```python
from build123d import *

# Parameters (mm, degrees)
SKETCH001_W          = 167.35
SKETCH001_H          = 77.5
SKETCH001_W_2        = 91
SKETCH001_H_2        = 58.3
PAD_DEPTH            = 2.5
SKETCH_R             = 1.58
POCKET_DEPTH         = 0.001
POCKET_DEPTH_BACK    = 2.501
SKETCH002_W          = 96.2
SKETCH002_H          = 62.3
SKETCH002_W_2        = 91
SKETCH002_H_2        = 58.3
PAD001_DEPTH         = 37
SKETCH003_W          = 96.2
SKETCH003_H          = 62.3
PAD002_DEPTH         = 1.5
SKETCH004_W          = 19.5
SKETCH004_H          = 21
POCKET001_DEPTH      = 9.601
SKETCH005_W          = 53.9
SKETCH005_H          = 37
POCKET002_DEPTH      = 48.5
SKETCH007_W          = 16
SKETCH007_H          = 11.1
SKETCH007_W_2        = 9.8
SKETCH007_H_2        = 8.8
POCKET003_DEPTH      = 38.751
FILLET_R             = 2
POCKET004_DEPTH      = 377.854265
POCKET004_DEPTH_BACK = 418.854265


with BuildPart() as part:
    # Sketch001 → Pad (new body)
    with BuildSketch(Plane.XY):
        Rectangle(SKETCH001_W, SKETCH001_H)
        Rectangle(SKETCH001_W_2, SKETCH001_H_2, mode=Mode.SUBTRACT)
    extrude(amount=PAD_DEPTH)

    # Sketch → Pocket (cut, two sides)
    with BuildSketch(Plane.XY) as pocket_sk:
        with Locations((-76.675, -31.75)):
            Circle(SKETCH_R)
        with Locations((-76.675, 31.75)):
            Circle(SKETCH_R)
        with Locations((76.675, 31.75)):
            Circle(SKETCH_R)
        with Locations((76.675, -31.75)):
            Circle(SKETCH_R)
    extrude(amount=-POCKET_DEPTH, mode=Mode.SUBTRACT)
    extrude(pocket_sk.sketch, amount=POCKET_DEPTH_BACK, mode=Mode.SUBTRACT)

    # Sketch002 → Pad001 (join)
    with BuildSketch(Plane.XY.offset(2.5)):
        with Locations((-0.4, 1)):
            Rectangle(SKETCH002_W, SKETCH002_H)
        Rectangle(SKETCH002_W_2, SKETCH002_H_2, mode=Mode.SUBTRACT)
    extrude(amount=PAD001_DEPTH)

    # Sketch003 → Pad002 (join)
    with BuildSketch(Plane.XY.offset(39.5)):
        with Locations((-0.4, 1)):
            Rectangle(SKETCH003_W, SKETCH003_H)
        with BuildLine():
            ThreePointArc((0, 11.892024), (-16.168632, 3.339331), (-18.197313, -14.839164))
            ThreePointArc((-18.197313, -14.839164), (-15.316051, -16.091394), (-14.063821, -13.210132))
            ThreePointArc((0, 7.449109), (-12.495952, 0.839146), (-14.063821, -13.210132))
            ThreePointArc((0, 7.449109), (2.221458, 9.670566), (0, 11.892024))
        make_face(mode=Mode.SUBTRACT)
        with BuildLine():
            ThreePointArc((-0.208963, -6.182796), (15.203911, -11.065575), (21.251521, 3.928579))
            ThreePointArc((25.403758, 5.50922), (22.537319, 6.795018), (21.251521, 3.928579))
            ThreePointArc((-4.071455, -8.378395), (17.097581, -15.084718), (25.403758, 5.50922))
            ThreePointArc((-0.208963, -6.182796), (-3.238008, -5.349349), (-4.071455, -8.378395))
        make_face(mode=Mode.SUBTRACT)
        with BuildLine():
            ThreePointArc((31.656498, 5.917571), (17.941279, 12.959928), (14.941672, -2.163047))
            ThreePointArc((11.627583, -5.122155), (14.764181, -5.299645), (14.941672, -2.163047))
            ThreePointArc((36.034044, 6.676909), (16.007515, 16.959935), (11.627583, -5.122155))
            ThreePointArc((31.656498, 5.917571), (34.22494, 4.108467), (36.034044, 6.676909))
        make_face(mode=Mode.SUBTRACT)
        with BuildLine():
            ThreePointArc((-4.63181, 21.445734), (-29.723459, 6.034298), (-24.464471, -22.938901))
            ThreePointArc((-24.464471, -22.938901), (-21.322913, -22.957951), (-21.303863, -19.816393))
            ThreePointArc((-4.849326, 17.008146), (-25.66708, 4.221761), (-21.303863, -19.816393))
            ThreePointArc((-4.849326, 17.008146), (-2.521774, 19.118182), (-4.63181, 21.445734))
        make_face(mode=Mode.SUBTRACT)
    extrude(amount=PAD002_DEPTH)

    # Sketch004 → Pocket001 (cut, through all)
    with BuildSketch(Plane.XZ.offset(-29.15)):
        with Locations((-40.015, 10.5)):
            Rectangle(SKETCH004_W, SKETCH004_H)
    extrude(amount=-POCKET001_DEPTH, mode=Mode.SUBTRACT)

    # Sketch005 → Pocket002 (cut)
    with BuildSketch(Plane.YZ):
        with Locations((0, 21)):
            Rectangle(SKETCH005_W, SKETCH005_H)
    extrude(amount=POCKET002_DEPTH, mode=Mode.SUBTRACT)

    # Sketch007 → Pocket003 (cut, through all)
    with BuildSketch(Plane(origin=(0, 0, 0), x_dir=(-1, 0, 0), z_dir=(0, 1, 0))):
        with BuildLine():
            Line((-15.6, 2.5), (-15.6, 10.1))
            ThreePointArc((-7.8, 10.1), (-11.7, 14), (-15.6, 10.1))
            Line((-7.8, 2.5), (-7.8, 10.1))
            Line((-15.6, 2.5), (-7.8, 2.5))
        make_face()
        with Locations((10.52, 8.05)):
            Rectangle(SKETCH007_W, SKETCH007_H)
        with Locations((32, 6.9)):
            Rectangle(SKETCH007_W_2, SKETCH007_H_2)
    extrude(amount=-POCKET003_DEPTH, mode=Mode.SUBTRACT)

    # Fillet
    fillet_edges = [part.edges().sort_by_distance(p)[0] for p in [
        (47.7, -30.15, 21),
        (47.7, 32.15, 21),
        (-48.5, 32.15, 30.25),
        (-48.5, -30.15, 21),
        (-83.675, -38.75, 1.25),
        (-83.675, 38.75, 1.25),
        (83.675, 38.75, 1.25),
        (83.675, -38.75, 1.25),
        (-49.765, 38.75, 1.25),
        (-30.265, 38.75, 1.25),
        (-45.5, 29.15, 1.25),
    ]]
    fillet(fillet_edges, radius=FILLET_R)

    # Sketch008 → Pocket004 (cut, two sides)
    with BuildSketch(Plane.XY) as pocket004_sk:
        with BuildLine():
            ThreePointArc((-56.80108, -10.00872), (-57.069005, 12.779324), (-77.692091, 22.477522))
            ThreePointArc((-77.692091, 22.477522), (-82.034221, 16.942851), (-76.49955, 12.60072))
            ThreePointArc((-65.292956, -4.82592), (-65.436679, 7.398302), (-76.49955, 12.60072))
            ThreePointArc((-65.292956, -4.82592), (-63.638418, -11.663258), (-56.80108, -10.00872))
        make_face()
        with BuildLine():
            ThreePointArc((-76.93054, -4.199269), (-74.278684, -23.506721), (-56.126644, -30.599921))
            ThreePointArc((-56.126644, -30.599921), (-53.792985, -27.379186), (-57.01372, -25.045527))
            ThreePointArc((-71.737576, -6.360594), (-69.860738, -20.025349), (-57.01372, -25.045527))
            ThreePointArc((-71.737576, -6.360594), (-73.253395, -2.68345), (-76.93054, -4.199269))
        make_face()
    pocket004 = extrude(amount=-POCKET004_DEPTH, mode=Mode.SUBTRACT) + extrude(pocket004_sk.sketch, amount=POCKET004_DEPTH_BACK, mode=Mode.SUBTRACT)

    # Mirrored: Pocket004 across Sketch008 V_Axis
    add(pocket004.mirror(Plane(origin=(0, 0, 0), x_dir=(0, 0, 1), z_dir=(1, 0, 0))), mode=Mode.SUBTRACT)


solid = part.part
```
Could you check a few things on this model? Use its own coordinates, in mm. A direction names the side the tool comes from. Round coordinates to 2 decimals unless told otherwise and drop trailing zeros. Loops run counter-clockwise (first coordinate to the right, second up) from the corner with the lowest first, then second, coordinate; pieces in that order, holes last. Notation, with made-up numbers: (-6.75, 76) -> (0.25, 76) arc R27 ccw to (0.25, 110) -> close; hole circle Ø11 at (-28.5, 60). An arc over 180 degrees is marked (long way). Put each result on its own line as item: value.
Q1. I want a section at B-B on x = -40. Write out the boundary of the cut face in (y, z), and give its area (3 significant figures).
Checks:
outline: (-38.75, 0) -> (-29.15, 0) -> (-29.15, 39.5) -> (29.15, 39.5) -> (29.15, 21) -> (32.15, 21) -> (32.15, 41) -> (-30.15, 41) -> (-30.15, 2.5) -> (-38.75, 2.5) -> close
area: 210 mm2
Q2. Which directions (+Z, -Z, +X, -X, +Y, -Y) give clear straight access to the entire face, cutting with the end or side of a thin tool? Please do faces 3 (the cylindrical face through (16.787, -15.227, 40.24)), 4 (the flat face through (-1, 29.15, 19)).
Checks:
face 3: +Z, -Z
face 4: -Z
Q3. For pin 1 Ø1.8 at (x, z) = (46, 13) entering from +Y; pin 2 Ø0.8 at (y, z) = (-30, 7.5) entering from -X; pin 3 Ø5 at (y, z) = (-3.5, 35.5) entering from -X; pin 4 Ø12 at (x, y) = (-45.5, 6) entering from -Z, each with a flat end and sliding along its axis, tell me the tip position at first contact or that it passes through.
Checks:
pin 1: y = 32.15
pin 2: x = -47.88
pin 3: x = -48.5
pin 4: z = 0
Q4. I want a section at A-A on z = 5. Give the number of separate pieces and of enclosed holes in the cut face, and give its area (3 significant figures).
Checks:
separate pieces: 5
enclosed holes: 0
area: 478 mm2
Q5. Please list where these lines run through material, in increasing order: line 1 (Z direction, x = 46.5, y = 4); line 2 (X direction, y = -31, z = 1) (3 decimals); line 3 (X direction, y = 31, z = 1) (3 decimals). Write a range as from..to.
Checks:
line 1: 0..2.5, 39.5..41
line 2: -83.675..-78.066, -75.284..75.284, 78.066..83.675
line 3: -83.675..-78.066, -75.284..-49.765, -30.265..75.284, 78.066..83.675
Q6. Thinking about a two-plate mould opening in Y: for faces 1 (the cylindrical face through (53.784, -27.44, 1.268)), 2 (the cylindrical face through (11.6, -29.6, 14)), which applies, pulls with the +Y half, pulls with the -Y half, needs draft (parallel to the pull), parting line crosses it, or undercut?
Checks:
face 1: undercut
face 2: needs draft
